```python
from build123d import *

# Parameters (mm, degrees)
F1_DEPTH = 25.4
F2_T     = -3.175
F3_DEPTH = 25.4
F4_R     = 3.175
F5_DEPTH = 3.175
F6_R     = 3.175
F7_DEPTH = 25.4
F9_DEPTH = 3.175


# Not quite as in the source:
# - a feature names something its author has since deleted; it is built from what else it names


with BuildPart() as f1:
    # F0 (on Top) → F1 (new body)
    with BuildSketch(Plane.XY):
        Polygon((11.90625, 11.90625), (-11.90625, 11.90625), (-11.90625, -11.90625), align=None)
    extrude(amount=F1_DEPTH)

    # F2
    f2_openings = [f1.faces().sort_by_distance(p)[0] for p in [
        (0, 11.90625, 12.7),
    ]]
    offset(amount=F2_T, openings=f2_openings)

    # F3 (cut): a face of the model
    f3_faces = [f1.faces().sort_by_distance(p)[0] for p in [
        (-3.3487926868, 6.5237926868, 3.175),
    ]]
    extrude(f3_faces, amount=-F3_DEPTH, mode=Mode.SUBTRACT)

    # F4 (on face) → F5 (cut)
    with BuildSketch(Plane(origin=(-11.90625, 0, 0), x_dir=(0, -1, 0), z_dir=(-1, 0, 0))):
        with Locations((-2.38125, 12.7)):
            Circle(F4_R)
    extrude(amount=-F5_DEPTH, mode=Mode.SUBTRACT)

    # F6 (on face) → F7 (cut)
    with BuildSketch(Plane.XY.offset(25.4)):
        with Locations((-2.38125, 7.46125)):
            Circle(F6_R)
    extrude(amount=-F7_DEPTH, mode=Mode.SUBTRACT)

    # F8 (on face) → F9 (cut)
    with BuildSketch(Plane(origin=(0, 0, 0), x_dir=(0.7071067812, 0.7071067812, 0), z_dir=(0.7071067812, -0.7071067812, 0))):
        with BuildLine():
            ThreePointArc((3.175, 12.7), (1.0081076412, 15.7107048982), (-2.5348229819, 14.6118832209))
            Line((-2.5348229819, 14.6118832209), (2.5348229819, 10.7881167791))
            ThreePointArc((2.5348229819, 10.7881167791), (3.0107048982, 11.6918923588), (3.175, 12.7))
        make_face()
        with BuildLine():
            Line((2.5348229819, 10.7881167791), (-2.5348229819, 14.6118832209))
            ThreePointArc((-2.5348229819, 14.6118832209), (-1.9118832209, 10.1651770181), (2.5348229819, 10.7881167791))
        make_face()
    extrude(amount=-F9_DEPTH, mode=Mode.SUBTRACT)


solid = f1.part
```
For this review, take the finished solid that the model builds, in its own axes (mm). A direction names the side the tool comes from. Give positions to 0.01 mm unless a question says otherwise; leave off trailing zeros. Write each loop counter-clockwise with the first axis right and the second up, starting at its lowest first coordinate (ties: lowest second). Pieces come first, ordered by that corner, then holes. Notation, with made-up numbers: M 31.5,-22 L 49.5,-22 A29 ccw 49.5,7 Z; hole C 40.25,46 d10. An arc over 180 degrees is marked long. One line per item, written item: value.
1) The part is to be moulded in two halves that separate along X. For faces 3 (the flat face through (-8.731, 6, 11)), 4 (the cylindrical face through (-10.34, 4.9, 10.77)), 5 (the flat face through (2.5, 2.5, 12.5)), say which applies: +X half, -X half, draft (parallel to the pull), parting line (faces both ways), or undercut.
Results are:
face 3: undercut
face 4: draft
face 5: +X half
2) Take a section at A-A, the plane z = 4. Write out the cut boundary in (x, y).
Results are:
outline: M -11.91,-11.91 L 11.91,11.91 L 7.42,11.91 L -8.73,-4.24 L -8.73,11.91 L -11.91,11.91 Z
3) Take a section at C-C, the plane x = -6. Write out the cut boundary in (y, z) (3 decimals).
Results are:
outline: M -6,0 L -1.51,0 L -1.51,22.225 L 11.906,22.225 L 11.906,25.4 L -6,25.4 Z
4) Take a section at B-B, the plane y = -8.5. Write out the cut boundary in (x, z), then the cut area to 3 significant figures.
Results are:
outline: M -11.91,0 L -8.5,0 L -8.5,25.4 L -11.91,25.4 Z
area: 86.5 mm²
5) Take a section at D-D, the plane x = 10. Write out the cut boundary in (y, z).
Results are:
outline: M 10,0 L 11.91,0 L 11.91,25.4 L 10,25.4 Z
6) For P1, Ø5, axis at y = 4, z = 10.5, coming from the +X side; P2, Ø8, axis at y = 8, z = 20, coming from the +X side; P3, Ø5, axis at y = -1, z = 8.5, coming from the +X side; P4, Ø10, axis at x = 4.5, y = -3.5, coming from the +Z side, all flat-tipped, find the tip position at first contact; note any pin that passes through.
Results are:
P1: stops at x = 6.5
P2: stops at x = 11.91
P3: stops at x = 1.5
P4: passes through
7) For line 1 (Z direction, x = -6.75, y = 3.25) (3 decimals); line 2 (X direction, y = 5.5, z = 3.5); line 3 (X direction, y = 7, z = 20), list the stretches that pass through material, from the lowest coordinate up. Write a range as from..to.
Results are:
line 1: z = 22.225..25.4
line 2: x = -11.91..-8.73, 1.01..5.5
line 3: x = -11.91..-8.73, 2.51..7
8) For faces 1 (the flat face through (-4, 0, 0)), 2 (the flat face through (-0.77, 3.72, 8.8)), list the 3-axis set-ups (+Z, -Z, +X, -X, +Y, -Y) from which the entire face can be reached by the end or side of a thin tool; tool diameter is ignored.
Results are:
face 1: -Z, +X, -X, +Y, -Y
face 2: -Z, +Y
